Verification items for the finished model (mm, model axes). Give positions to 0.01 mm unless a question says otherwise; leave off trailing zeros. Write each loop counter-clockwise with the first axis right and the second up, starting at its lowest first coordinate (ties: lowest second). Pieces come first, ordered by that corner, then holes.
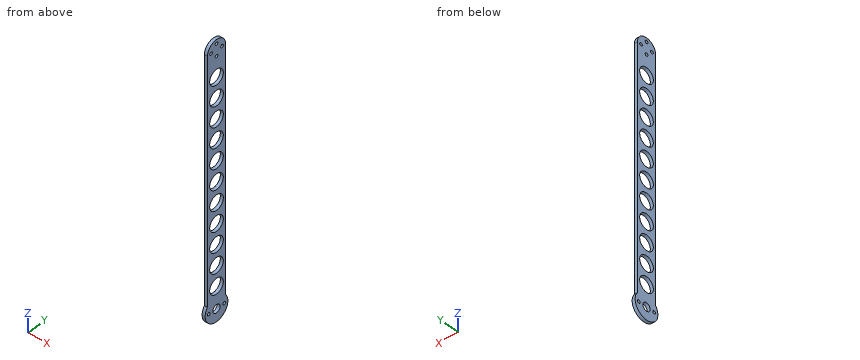
from build123d import *

# Parameters (mm, degrees)
EXTRUDE_1_DEPTH     = 3
SKETCH_2_R          = 1.5
SKETCH_2_R_2        = 4
CUT_EXTRUDE_1_DEPTH = 3
SKETCH_4_R          = 7.5
CUT_EXTRUDE_2_DEPTH = 250


with BuildPart() as part:
    # 草图1 → 凸台-拉伸1 (new body)
    with BuildSketch(Plane(origin=(0, 0, 0), x_dir=(0, 0, -1), z_dir=(1, 0, 0))):
        with BuildLine():
            Line((-120, 10), (120, 10))
            ThreePointArc((120, 10), (140, 0), (120, -10))
            Line((120, -10), (-120, -10))
            ThreePointArc((-120, -10), (-130.000001885, 0), (-120, 10))
        make_face()
    extrude(amount=EXTRUDE_1_DEPTH)

    # 草图2 → 切除-拉伸1 (cut)
    with BuildSketch(Plane(origin=(3, 0, 0), x_dir=(0, 0, -1), z_dir=(1, 0, 0))):
        with Locations((-120, 6)):
            Circle(SKETCH_2_R)
        with Locations((-114, 0)):
            Circle(SKETCH_2_R)
        with Locations((-120, -6)):
            Circle(SKETCH_2_R)
        with Locations((-126, 0)):
            Circle(SKETCH_2_R)
        with Locations((127.5, 8.5)):
            Circle(SKETCH_2_R)
        with Locations((127.5, -8.5)):
            Circle(SKETCH_2_R)
        with Locations((127.5, 0)):
            Circle(SKETCH_2_R_2)
    extrude(amount=-CUT_EXTRUDE_1_DEPTH, mode=Mode.SUBTRACT)

    # 草图4 → 切除-拉伸2 (cut)
    with BuildSketch(Plane(origin=(3, 0, 0), x_dir=(0, 0, -1), z_dir=(1, 0, 0))):
        with Locations((-94, 0)):
            Circle(SKETCH_4_R)
        with Locations((-74, 0)):
            Circle(SKETCH_4_R)
        with Locations((-54, 0)):
            Circle(SKETCH_4_R)
        with Locations((-34, 0)):
            Circle(SKETCH_4_R)
        with Locations((-14, 0)):
            Circle(SKETCH_4_R)
        with Locations((6, 0)):
            Circle(SKETCH_4_R)
        with Locations((26, 0)):
            Circle(SKETCH_4_R)
        with Locations((46, 0)):
            Circle(SKETCH_4_R)
        with Locations((66, 0)):
            Circle(SKETCH_4_R)
        with Locations((86, 0)):
            Circle(SKETCH_4_R)
        with Locations((106, 0)):
            Circle(SKETCH_4_R)
    extrude(amount=-CUT_EXTRUDE_2_DEPTH, mode=Mode.SUBTRACT)


solid = part.part
Item 1: Depth check by flat-ended pin: pin 1 (2.5 mm diameter, centred on y = 8.5, z = -127.5, fed in from -X); pin 2 (1.5 mm diameter, centred on x = 2.5, z = 40, fed in from +Y); pin 3 (1 mm diameter, centred on x = 1.5, y = -6.5, fed in from +Z). Enter the tip coordinate at first touch or a pass-through.
Answer key:
pin 1: passes through
pin 2: stops at y = 10
pin 3: stops at z = 128
Item 2: Sectioned sample at C-C on z = -65.5. Record the cut outline in (x, y).
Answer key:
outline: (0, -10) - (3, -10) - (3, -7.48) - (0, -7.48) - close; (0, 7.48) - (3, 7.48) - (3, 10) - (0, 10) - close
Item 3: Scan lines: line 1 along Y through (x, z) = (0.7, 120); line 2 along Y through (x, z) = (2.35, 14); line 3 along Z through (x, y) = (2.6, 7.75). Record each from-to range of solid material in increasing order.
Answer key:
line 1: y = -10 to -7.5, -4.5 to 4.5, 7.5 to 10
line 2: y = -10 to -7.5, 7.5 to 10
line 3: z = -137.31 to -128.8, -126.2 to 126.32
Item 4: Sectioned sample at A-A on z = -106. Record the cut outline in (x, y), then the cut area to 3 significant figures.
Answer key:
outline: (0, -10) - (3, -10) - (3, -7.5) - (0, -7.5) - close; (0, 7.5) - (3, 7.5) - (3, 10) - (0, 10) - close
area: 15.0 mm2
Item 5: Sectioned sample at B-B on x = 2.05. State how many separate pieces and enclosed holes the cut face has, then the cut area to 3 significant figures.
Answer key:
separate pieces: 1
enclosed holes: 18
area: 3,340 mm2
